Drawing for the job (mm, zero at the part's lowest x, y, z). A direction names the side the tool comes from. Coordinates: 2 decimals unless noted, no trailing zeros. Write each loop counter-clockwise with the first axis right and the second up, starting at its lowest first coordinate (ties: lowest second). Pieces come first, ordered by that corner, then holes. Notation, with made-up numbers: (-32, -17.75) -> (-4, -17.75) arc R16 ccw to (-4, -11.75) -> close; hole circle Ø5 at (71.5, 56.5). An arc over 180 degrees is marked (long way). Answer as CSV lines item,"result".
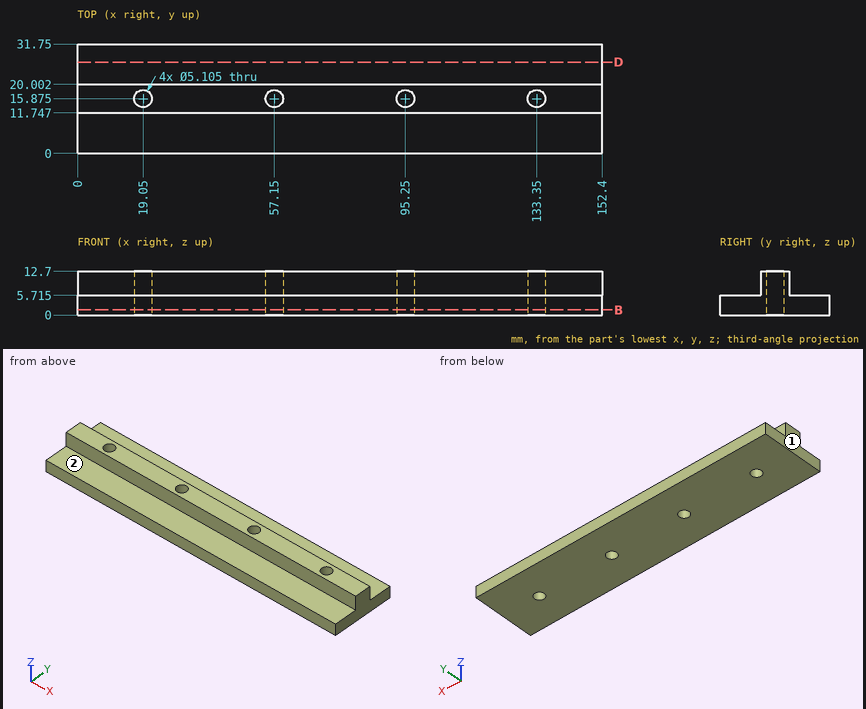
Item 1: Saw through at B-B on z = 1.5. State how many separate pieces and enclosed holes the cut face has, and give its area (3 significant figures).
Answer below:
separate pieces,"1"
enclosed holes,"4"
area,"4,760 mm2"
Item 2: Saw through at D-D on y = 26.5. Give the cut face in (x, z) (1 decimal).
Answer below:
outline,"(0, 0) -> (152.4, 0) -> (152.4, 5.7) -> (0, 5.7) -> close"
Item 3: 3-axis set-ups, long thin cutter, end or side, ignore diameter. For the marked faces 1 and 2: which of +Z, -Z, +X, -X, +Y, -Y reach the whole face in a straight line?
Answer below:
face 1,"+Z, -Z, -X, +Y, -Y"
face 2,"+Z, +X, -X, -Y"
Item 4: Wall check: line 1 (X direction, y = 14, z = 1.75) (1 decimal); line 2 (Y direction, x = 95.25, z = 3.5); line 3 (Y direction, x = 19.05, z = 8.5). Give the ranges that are in metal, low to high. Write a range as from..to.
Answer below:
line 1,"x = 0..17.3, 20.8..55.4, 58.9..93.5, 97..131.6, 135.1..152.4"
line 2,"y = 0..13.32, 18.43..31.75"
line 3,"y = 11.75..13.32, 18.43..20"
Item 5: Flat gauge pins, fed straight in: pin 1 (4 mm diameter, centred on x = 24.5, y = 8.5, fed in from +Z) (1 decimal); pin 2 (2 mm diameter, centred on x = 76, z = 8.5, fed in from +Y); pin 3 (2 mm diameter, centred on x = 91, z = 9, fed in from -Y). Where does each tip first touch, or does it go through?
Answer below:
pin 1,"stops at z = 5.7"
pin 2,"stops at y = 20"
pin 3,"stops at y = 11.75"
